Can you work these out from the drawing? Everything is in mm from the part's minimum corner. A direction names the side the tool comes from. Coordinates: 2 decimals unless noted, no trailing zeros. Loops run counter-clockwise (first coordinate to the right, second up) from the corner with the lowest first, then second, coordinate; pieces in that order, holes last.
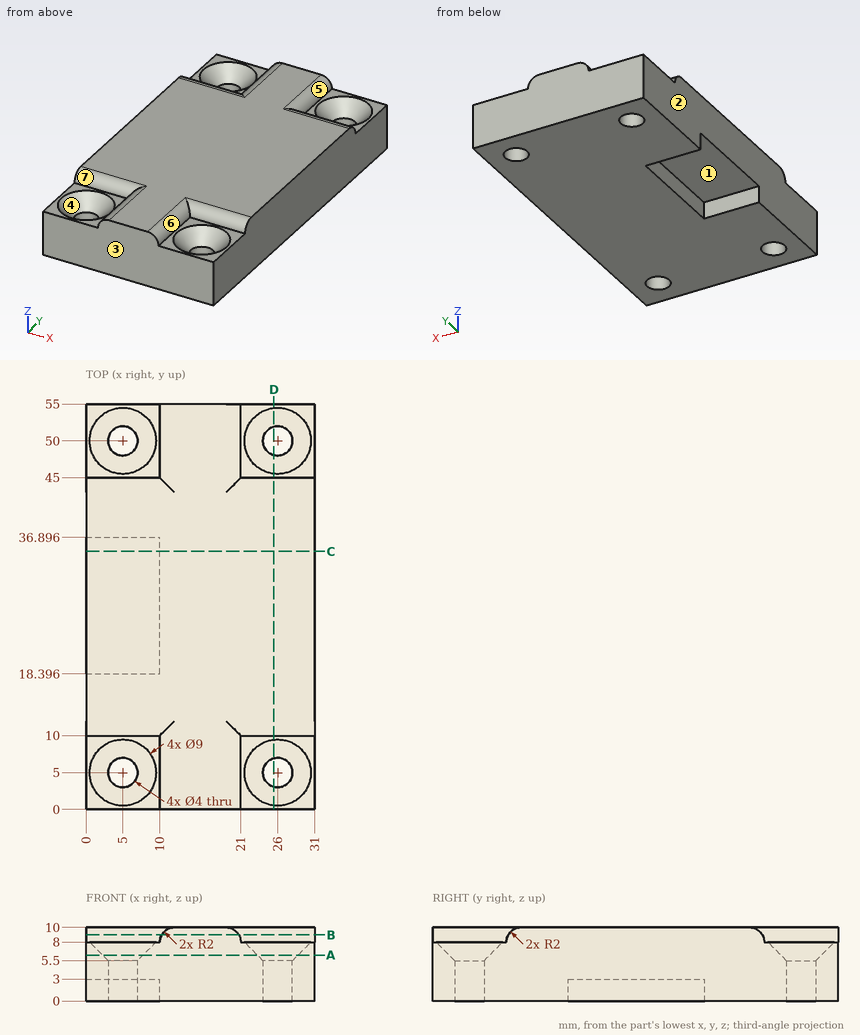
1) Imagine slicing it at C-C on y = 35. List the corners of the cut face in (x, z) for me, plus the area to 3 significant figures.
2) For the marked faces 5, 6 and 7, which set-ups out of +Z, -Z, +X, -X, +Y, -Y let a thin tool reach every point of the face, with its end or its side?
3) Imagine slicing it at B-B on z = 9. List the corners of the cut face in (x, y) for me.
4) If I drill on L1, parallel to X at y = 50, z = 5.5; L2, parallel to Y at x = 5, z = 4.75; L3, parallel to Y at x = 27, z = 4.75, over which ranges is the centre line in solid material (lowest first)?
5) Will these pins go through, and if not, where does the flat tip stop? pin 1 (3 mm diameter, centred on x = 7.5, y = 47.5, fed in from +Z); pin 2 (2.5 mm diameter, centred on x = 26, y = 5, fed in from +Z); pin 3 (8 mm diameter, centred on x = 23.5, y = 48.5, fed in from +Z); pin 4 (1.5 mm diameter, centred on y = 25.5, z = 1.5, fed in from -X).
6) Imagine slicing it at A-A on z = 6.25. List the corners of the cut face in (x, y) for me.
7) Imagine slicing it at D-D on x = 25.5. State how many separate pieces and enclosed holes the cut face has, plus the area to 3 significant figures.
8) We'd pull the mould along Y, two halves only. Please class the marked faces 1, 2, 3 and 4: released by +Y, released by -Y, zero draft, split by the parting line, or undercut.
Solved:
1. outline: (0, 3) - (10, 3) - (10, 0) - (31, 0) - (31, 10) - (0, 10) - close
1. area: 280 mm2
2. face 5: +Z, +X, +Y
2. face 6: +Z, +X, -Y
2. face 7: +Z, -X, -Y
3. outline: (0, 10.27) - (10.27, 10.27) - (10.27, 0) - (20.73, 0) - (20.73, 10.27) - (31, 10.27) - (31, 44.73) - (20.73, 44.73) - (20.73, 55) - (10.27, 55) - (10.27, 44.73) - (0, 44.73) - close
4. L1: x = 0 to 3, 7 to 24, 28 to 31
4. L2: y = 0 to 3, 7 to 48, 52 to 55
4. L3: y = 0 to 3.27, 6.73 to 48.27, 51.73 to 55
5. pin 1: stops at z = 8
5. pin 2: passes through
5. pin 3: stops at z = 9.94
5. pin 4: stops at x = 10
6. outline: (0, 0) - (31, 0) - (31, 55) - (0, 55) - close; hole circle Ø5.5 at (5, 5); hole circle Ø5.5 at (5, 50); hole circle Ø5.5 at (26, 5); hole circle Ø5.5 at (26, 50)
7. separate pieces: 3
7. enclosed holes: 0
7. area: 434 mm2
8. face 1: undercut
8. face 2: zero draft
8. face 3: released by -Y
8. face 4: undercut
